Geometry: final body of the model. Coordinates: model frame, mm. Give positions to 0.01 mm unless a question says otherwise; leave off trailing zeros. Write each loop counter-clockwise with the first axis right and the second up, starting at its lowest first coordinate (ties: lowest second). Pieces come first, ordered by that corner, then holes. Notation, with made-up numbers: (60.25, 17.25) - (110.25, 17.25) arc R21 cw to (110.25, 44.25) - close; hole circle Ø3 at (7, 8). An arc over 180 degrees is marked (long way). Use CSV: the item, a comma, the result in double quotes. Start each with the question number.
(1) Line query: probe 1 along X at (y, z) = (2.15, 18.5); probe 2 along X at (y, z) = (4.7, -1); probe 3 along Z at (x, y) = (12, 3.5). Output: solid intervals per line, ascending. Write a range as [from, to].
(2) Section A-A on x = 0. Output: boundary loops of the cut face in (y, z), and give its area (3 significant figures).
(3) Section D-D on y = 4.5. Count the separate pieces of the cut face and the enclosed holes in it, and give its area (3 significant figures).
(4) Section B-B on z = 0. Output: boundary loops of the cut face in (x, y), and give its area (3 significant figures).
(5) Draft query along X for faces 1 (the cylindrical face through (-48.89, 2.96, -10.86)), 2 (the cylindrical face through (19.4, 2.96, 34.11)), 3 (the flat face through (1, 0, 10)). Return one class per face: released by +X, released by -X, zero draft, split by the parting line, or undercut.
(6) First-contact query: pin 1 Ø1.5 at (y, z) = (4, -13.5) entering from +X; pin 2 Ø3 at (x, y) = (-20, 4) entering from +Z; pin 3 Ø1 at (x, y) = (18, 3) entering from -Z. Flat tips, straight axial feed; report the tip coordinate or a pass-through.
(7) Section C-C on z = -38.1. Output: boundary loops of the cut face in (x, y), and give its area (3 significant figures).
from build123d import *

# Parameters (mm, degrees)
SKETCH1_R           = 50
SKETCH1_R_2         = 1.25
SKETCH1_R_3         = 1.5
SKETCH1_R_4         = 4
BOSS_EXTRUDE1_DEPTH = 6
MOVE_FACE1_BY       = 0.08
MOVE_FACE1_2_BY     = 0.08
MOVE_FACE1_3_BY     = 0.08
MOVE_FACE1_4_BY     = 0.08
MOVE_FACE1_5_BY     = 0.08
MOVE_FACE1_6_BY     = 0.08
MOVE_FACE1_7_BY     = 0.08
MOVE_FACE1_8_BY     = 0.08
MOVE_FACE1_9_BY     = 0.08
MOVE_FACE1_10_BY    = 0.08
MOVE_FACE1_11_BY    = 0.08
MOVE_FACE1_12_BY    = 0.08
MOVE_FACE1_13_BY    = 0.08
MOVE_FACE1_14_BY    = 0.08


with BuildPart() as part:
    # Sketch1 → Boss-Extrude1 (new body)
    with BuildSketch(Plane(origin=(0, 0, 0), x_dir=(1, 0, 0), z_dir=(0, 1, 0))):
        with Locations(Location((0, 0, 0), (0, 0, 270))):
            Circle(SKETCH1_R)
        with Locations(Location((38.1, 0, 0), (0, 0, 270))):
            Circle(SKETCH1_R_2, mode=Mode.SUBTRACT)
        with Locations(Location((19.05, -32.995567884, 0), (0, 0, 270))):
            Circle(SKETCH1_R_2, mode=Mode.SUBTRACT)
        with Locations(Location((-19.05, -32.995567884, 0), (0, 0, 270))):
            Circle(SKETCH1_R_2, mode=Mode.SUBTRACT)
        with Locations(Location((-38.1, 0, 0), (0, 0, 270))):
            Circle(SKETCH1_R_2, mode=Mode.SUBTRACT)
        with Locations(Location((-19.05, 32.995567884, 0), (0, 0, 270))):
            Circle(SKETCH1_R_2, mode=Mode.SUBTRACT)
        with Locations(Location((19.05, 32.995567884, 0), (0, 0, 270))):
            Circle(SKETCH1_R_2, mode=Mode.SUBTRACT)
        with Locations(Location((0, 38.1, 0), (0, 0, 270))):
            Circle(SKETCH1_R_3, mode=Mode.SUBTRACT)
        with Locations(Location((32.995567884, 19.05, 0), (0, 0, 270))):
            Circle(SKETCH1_R_3, mode=Mode.SUBTRACT)
        with Locations(Location((32.995567884, -19.05, 0), (0, 0, 270))):
            Circle(SKETCH1_R_3, mode=Mode.SUBTRACT)
        with Locations(Location((0, -38.1, 0), (0, 0, 270))):
            Circle(SKETCH1_R_3, mode=Mode.SUBTRACT)
        with Locations(Location((-32.995567884, -19.05, 0), (0, 0, 270))):
            Circle(SKETCH1_R_3, mode=Mode.SUBTRACT)
        with Locations(Location((-32.995567884, 19.05, 0), (0, 0, 270))):
            Circle(SKETCH1_R_3, mode=Mode.SUBTRACT)
        with Locations(Location((0, 0, 0), (0, 0, 270))):
            Circle(SKETCH1_R_4, mode=Mode.SUBTRACT)
    extrude(amount=BOSS_EXTRUDE1_DEPTH)

    # Move Face1: a curved face moved outward by 0.08
    add(Solid.thicken(part.faces().sort_by_distance((0, 3, -4))[0], MOVE_FACE1_BY))

    # Move Face1 2: a curved face moved outward by 0.08
    add(Solid.thicken(part.faces().sort_by_distance((0, 3, -50))[0], MOVE_FACE1_2_BY))

    # Move Face1 3: a curved face moved outward by 0.08
    add(Solid.thicken(part.faces().sort_by_distance((38.1, 3, -1.25))[0], MOVE_FACE1_3_BY))

    # Move Face1 4: a curved face moved outward by 0.08
    add(Solid.thicken(part.faces().sort_by_distance((0, 3, -39.6))[0], MOVE_FACE1_4_BY))

    # Move Face1 5: a curved face moved outward by 0.08
    add(Solid.thicken(part.faces().sort_by_distance((19.05, 3, 31.745567884))[0], MOVE_FACE1_5_BY))

    # Move Face1 6: a curved face moved outward by 0.08
    add(Solid.thicken(part.faces().sort_by_distance((-19.05, 3, 31.745567884))[0], MOVE_FACE1_6_BY))

    # Move Face1 7: a curved face moved outward by 0.08
    add(Solid.thicken(part.faces().sort_by_distance((-38.1, 3, -1.25))[0], MOVE_FACE1_7_BY))

    # Move Face1 8: a curved face moved outward by 0.08
    add(Solid.thicken(part.faces().sort_by_distance((-19.05, 3, -34.245567884))[0], MOVE_FACE1_8_BY))

    # Move Face1 9: a curved face moved outward by 0.08
    add(Solid.thicken(part.faces().sort_by_distance((19.05, 3, -34.245567884))[0], MOVE_FACE1_9_BY))

    # Move Face1 10: a curved face moved outward by 0.08
    add(Solid.thicken(part.faces().sort_by_distance((32.995567884, 3, -20.55))[0], MOVE_FACE1_10_BY))

    # Move Face1 11: a curved face moved outward by 0.08
    add(Solid.thicken(part.faces().sort_by_distance((32.995567884, 3, 17.55))[0], MOVE_FACE1_11_BY))

    # Move Face1 12: a curved face moved outward by 0.08
    add(Solid.thicken(part.faces().sort_by_distance((0, 3, 36.6))[0], MOVE_FACE1_12_BY))

    # Move Face1 13: a curved face moved outward by 0.08
    add(Solid.thicken(part.faces().sort_by_distance((-32.995567884, 3, 17.55))[0], MOVE_FACE1_13_BY))

    # Move Face1 14: a curved face moved outward by 0.08
    add(Solid.thicken(part.faces().sort_by_distance((-32.995567884, 3, -20.55))[0], MOVE_FACE1_14_BY))


solid = part.part
Check values:
1,probe 1,"x = [-46.54, -34.3], [-31.69, 31.69], [34.3, 46.54]"
1,probe 2,"x = [-50.07, -38.71], [-37.49, -3.79], [3.79, 37.49], [38.71, 50.07]"
1,probe 3,"z = [-48.62, 48.62]"
2,outline,"(0, -50.08) - (6, -50.08) - (6, -39.52) - (0, -39.52) - close; (0, -36.68) - (6, -36.68) - (6, -3.92) - (0, -3.92) - close; (0, 3.92) - (6, 3.92) - (6, 36.68) - (0, 36.68) - close; (0, 39.52) - (6, 39.52) - (6, 50.08) - (0, 50.08) - close"
2,area,"520 mm²"
3,separate pieces,"1"
3,enclosed holes,"13"
3,area,"7,770 mm²"
4,outline,"(-50.08, 0) - (-39.27, 0) - (-39.27, 6) - (-50.08, 6) - close; (-36.93, 0) - (-3.92, 0) - (-3.92, 6) - (-36.93, 6) - close; (3.92, 0) - (36.93, 0) - (36.93, 6) - (3.92, 6) - close; (39.27, 0) - (50.08, 0) - (50.08, 6) - (39.27, 6) - close"
4,area,"526 mm²"
5,face 1,"split by the parting line"
5,face 2,"undercut"
5,face 3,"zero draft"
6,pin 1,"stops at x = 48.43"
6,pin 2,"stops at z = 46.54"
6,pin 3,"stops at z = -46.92"
7,outline,"(-32.5, 0) - (-1.42, 0) - (-1.42, 6) - (-32.5, 6) - close; (1.42, 0) - (32.5, 0) - (32.5, 6) - (1.42, 6) - close"
7,area,"373 mm²"
